CAD build for the part. Positions are in the model's coordinates, mm. Coordinates: 2 decimals unless noted, no trailing zeros. Loops run counter-clockwise (first coordinate to the right, second up) from the corner with the lowest first, then second, coordinate; pieces in that order, holes last.
1) Pin check, flat tips, straight feed: pin 1 Ø6.5 at (x, z) = (-201.5, -35) entering from +Y; pin 2 Ø4 at (y, z) = (10.5, -1) entering from -X; pin 3 Ø6.5 at (y, z) = (13.5, -61) entering from +X. Stop position of each tip, or through.
2) Saw through at C-C, the plane x = -180.5. Write the cut outline in (y, z), and give its area (3 significant figures).
3) Saw through at B-B, the plane y = 12. Write the cut outline in (x, z).
4) Wall check: line 1 along X through (y, z) = (17, 64.5) (1 decimal); line 2 along X through (y, z) = (15, -109); line 3 along Z through (x, y) = (148, 10.5). Give the ranges that are in metal, low to high.
```python
from build123d import *

# Parameters (mm, degrees)
SKETCH1_W           = 422.275
SKETCH1_H           = 241.3
BOSS_EXTRUDE1_DEPTH = 19.05
CUT_EXTRUDE1_REACH  = 323.197
SKETCH2_W           = 13.49375
SKETCH2_H           = 3.175
SKETCH2_W_2         = 14.2875
FILLET1_R           = 63.5
CUT_EXTRUDE2_REACH  = 323.197
SKETCH3_W           = 13.49375
SKETCH3_H           = 9.525


with BuildPart() as part:
    # Sketch1 → Boss-Extrude1 (new body)
    with BuildSketch(Plane(origin=(0, 0, 0), x_dir=(1, 0, 0), z_dir=(0, 1, 0))):
        Rectangle(SKETCH1_W, SKETCH1_H)
    extrude(amount=BOSS_EXTRUDE1_DEPTH)

    # Sketch2 → Cut-Extrude1 (cut, up to next)
    with BuildSketch(Plane.XY.offset(120.65), mode=Mode.PRIVATE) as cut_extrude1_sk1:
        with Locations((-204.390625, 17.4625)):
            Rectangle(SKETCH2_W, SKETCH2_H)
    cut_extrude1_tool1 = extrude(cut_extrude1_sk1.sketch, amount=-CUT_EXTRUDE1_REACH, mode=Mode.PRIVATE) & part.part
    # Sketch2 → Cut-Extrude1 (cut, up to next)
    with BuildSketch(Plane.XY.offset(120.65), mode=Mode.PRIVATE) as cut_extrude1_sk2:
        with Locations((-123.03125, 17.4625)):
            Rectangle(SKETCH2_W_2, SKETCH2_H)
    cut_extrude1_tool2 = extrude(cut_extrude1_sk2.sketch, amount=-CUT_EXTRUDE1_REACH, mode=Mode.PRIVATE) & part.part
    # Sketch2 → Cut-Extrude1 (cut, up to next)
    with BuildSketch(Plane.XY.offset(120.65), mode=Mode.PRIVATE) as cut_extrude1_sk3:
        with Locations((123.03125, 17.4625)):
            Rectangle(SKETCH2_W_2, SKETCH2_H)
    cut_extrude1_tool3 = extrude(cut_extrude1_sk3.sketch, amount=-CUT_EXTRUDE1_REACH, mode=Mode.PRIVATE) & part.part
    # Sketch2 → Cut-Extrude1 (cut, up to next)
    with BuildSketch(Plane.XY.offset(120.65), mode=Mode.PRIVATE) as cut_extrude1_sk4:
        with Locations((204.390625, 17.4625)):
            Rectangle(SKETCH2_W, SKETCH2_H)
    cut_extrude1_tool4 = extrude(cut_extrude1_sk4.sketch, amount=-CUT_EXTRUDE1_REACH, mode=Mode.PRIVATE) & part.part
    add(cut_extrude1_tool1.solids().sort_by_distance((-204.390625, 17.4625, 120.65))[0], mode=Mode.SUBTRACT)
    add(cut_extrude1_tool2.solids().sort_by_distance((-123.03125, 17.4625, 120.65))[0], mode=Mode.SUBTRACT)
    add(cut_extrude1_tool3.solids().sort_by_distance((123.03125, 17.4625, 120.65))[0], mode=Mode.SUBTRACT)
    add(cut_extrude1_tool4.solids().sort_by_distance((204.390625, 17.4625, 120.65))[0], mode=Mode.SUBTRACT)

    # Fillet1
    fillet1_edges = [part.edges().sort_by_distance(p)[0] for p in [
        (211.1375, 7.9375, 120.65),
        (-211.1375, 7.9375, 120.65),
    ]]
    fillet(fillet1_edges, radius=FILLET1_R)

    # Sketch3 → Cut-Extrude2 (cut, up to next)
    with BuildSketch(Plane(origin=(0, 0, -120.65), x_dir=(-1, 0, 0), z_dir=(0, 0, -1)), mode=Mode.PRIVATE) as cut_extrude2_sk1:
        with Locations((-204.390625, 11.1125)):
            Rectangle(SKETCH3_W, SKETCH3_H)
    cut_extrude2_tool1 = extrude(cut_extrude2_sk1.sketch, amount=-CUT_EXTRUDE2_REACH, mode=Mode.PRIVATE) & part.part
    # Sketch3 → Cut-Extrude2 (cut, up to next)
    with BuildSketch(Plane(origin=(0, 0, -120.65), x_dir=(-1, 0, 0), z_dir=(0, 0, -1)), mode=Mode.PRIVATE) as cut_extrude2_sk2:
        with Locations((204.390625, 11.1125)):
            Rectangle(SKETCH3_W, SKETCH3_H)
    cut_extrude2_tool2 = extrude(cut_extrude2_sk2.sketch, amount=-CUT_EXTRUDE2_REACH, mode=Mode.PRIVATE) & part.part
    add(cut_extrude2_tool1.solids().sort_by_distance((204.390625, 11.1125, -120.65))[0], mode=Mode.SUBTRACT)
    add(cut_extrude2_tool2.solids().sort_by_distance((-204.390625, 11.1125, -120.65))[0], mode=Mode.SUBTRACT)


solid = part.part
```
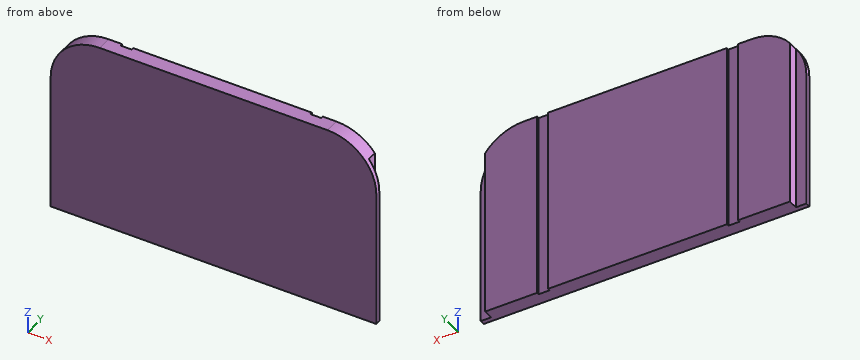
Data:
1. pin 1: stops at y = 6.35
1. pin 2: stops at x = -197.64
1. pin 3: stops at x = 197.64
2. outline: (0, -120.65) - (19.05, -120.65) - (19.05, 111.49) - (0, 111.49) - close
2. area: 4,420 mm2
3. outline: (-197.64, -120.65) - (197.64, -120.65) - (197.64, 96.29) arc R63.5 ccw to (147.64, 120.65) - (-147.64, 120.65) arc R63.5 ccw to (-197.64, 96.29) - close
4. line 1: x = -197.6 to -130.2, -115.9 to 115.9, 130.2 to 197.6
4. line 2: x = -197.64 to 197.64
4. line 3: z = -120.65 to 120.65
